```python
from build123d import *

# Parameters (mm, degrees)
SKETCH1_W               = 30.48
SKETCH1_H               = 25.4
BOSS_EXTRUDE1_DEPTH     = 30.48
SKETCH5_W               = 6.35
SKETCH5_H               = 28.956
CUT_EXTRUDE4_DEPTH      = 47.117696394
CUT_EXTRUDE5_DEPTH      = 40.787452235
CUT_EXTRUDE5_DEPTH_BACK = 40.787452235
SKETCH7_W               = 6.35
SKETCH7_H               = 1.524
CUT_EXTRUDE6_DEPTH      = 31.75


with BuildPart() as part:
    # Sketch1 → Boss-Extrude1 (new body)
    with BuildSketch(Plane(origin=(0, 0, 0), x_dir=(1, 0, 0), z_dir=(0, 1, 0))):
        with Locations((-4.387272727, -3.694545455)):
            Rectangle(SKETCH1_W, SKETCH1_H)
    extrude(amount=BOSS_EXTRUDE1_DEPTH)

    # Sketch5 → Cut-Extrude4 (cut, through all)
    with BuildSketch(Plane(origin=(10.852727273, 0, 0), x_dir=(0, 0, -1), z_dir=(1, 0, 0))):
        with Locations((-13.219545455, 16.002)):
            Rectangle(SKETCH5_W, SKETCH5_H)
        with Locations((5.830454545, 16.002)):
            Rectangle(SKETCH5_W, SKETCH5_H)
    extrude(amount=-CUT_EXTRUDE4_DEPTH, mode=Mode.SUBTRACT)

    # Sketch6 → Cut-Extrude5 (cut, two sides: drawn at the far end of the back side and taken through both)
    with BuildSketch(Plane.XY.offset(-CUT_EXTRUDE5_DEPTH_BACK)):
        Polygon((-18.103272727, 0), (-18.103272727, 28.956), (9.328727273, 28.956), (9.328727273, 1.524), (-8.342365858, 1.524), (-8.342365858, 0), align=None)
    extrude(amount=CUT_EXTRUDE5_DEPTH + CUT_EXTRUDE5_DEPTH_BACK, mode=Mode.SUBTRACT)

    # Sketch7 → Cut-Extrude6 (cut)
    with BuildSketch(Plane(origin=(-18.103272727, 0, 0), x_dir=(0, 0, -1), z_dir=(1, 0, 0))):
        with Locations((-13.219545455, 0.762)):
            Rectangle(SKETCH7_W, SKETCH7_H)
        with Locations((5.830454545, 0.762)):
            Rectangle(SKETCH7_W, SKETCH7_H)
    extrude(amount=-CUT_EXTRUDE6_DEPTH, mode=Mode.SUBTRACT)


solid = part.part
```
Design review of the part built by this model. Coordinates are the model's own, in mm. A direction names the side the tool comes from. Coordinates: 2 decimals unless noted, no trailing zeros. Order: outer loops, then holes, each group sorted by start corner. A loop starts at its lowest first (then second) coordinate and runs counter-clockwise, first axis right, second up.
1) Take a section at A-A, the plane y = 4. Give the boundary of the cut face in (x, z), and give its area (3 significant figures).
2) Clearance check with a flat-ended pin moving along its axis: pin 1 (5 mm diameter, centred on x = -16, y = 4.5, fed in from -Z). State where the tip first meets the part, or that it passes through.
3) Take a section at B-B, the plane x = -6.5. Give the boundary of the cut face in (y, z), and give its area (3 significant figures).
4) Wall thickness on line 1 along X through (y, z) = (3, 0.75); line 2 along Y through (x, z) = (-2, -1.5); line 3 along Y through (x, z) = (0, -2.75): over which ranges is each line inside the solid? List them lowest first.
5) For faces 1 (the flat face through (-5, 28.956, 4)), 2 (the flat face through (1, 1, 16.395)), 3 (the flat face through (-8.342, 1, 4)), list the 3-axis set-ups (+Z, -Z, +X, -X, +Y, -Y) from which the entire face can be reached by the end or side of a thin tool; tool diameter is ignored.
6) Mouldability with a two-part tool opening along X and no side actions: class faces 4 (the flat face through (10.853, 15, 4)), 5 (the flat face through (9.329, 15, 4)), 6 (the flat face through (1, 0, 4)), 7 (the flat face through (-19.627, 15, 4)) as +X half, -X half, draft (parallel to the pull), parting line (faces both ways), or undercut.
7) Take a section at C-C, the plane z = -1.5. Give the boundary of the cut face in (x, y).
8) Take a section at D-D, the plane x = -14. Give the boundary of the cut face in (y, z).
Returned:
1. outline: (-19.63, -2.66) - (-18.1, -2.66) - (-18.1, 10.04) - (-19.63, 10.04) - close; (9.33, -2.66) - (10.85, -2.66) - (10.85, 10.04) - (9.33, 10.04) - close
1. area: 38.7 mm2
2. pin 1: stops at z = -2.66
3. outline: (0, -9.01) - (1.52, -9.01) - (1.52, 16.39) - (0, 16.39) - close; (28.96, -2.66) - (30.48, -2.66) - (30.48, 10.04) - (28.96, 10.04) - close
3. area: 58.1 mm2
4. line 1: x = -19.63 to -18.1, 9.33 to 10.85
4. line 2: y = 0 to 1.52, 28.96 to 30.48
4. line 3: y = 0 to 1.52
5. face 1: +Z, -Z
5. face 2: +Z, +X, -X, +Y, -Y
5. face 3: +Z, -Z, -Y
6. face 4: +X half
6. face 5: undercut
6. face 6: draft
6. face 7: -X half
7. outline: (-19.63, 0) - (-18.1, 0) - (-18.1, 28.96) - (9.33, 28.96) - (9.33, 1.52) - (-8.34, 1.52) - (-8.34, 0) - (10.85, 0) - (10.85, 30.48) - (-19.63, 30.48) - close
8. outline: (28.96, -2.66) - (30.48, -2.66) - (30.48, 10.04) - (28.96, 10.04) - close
